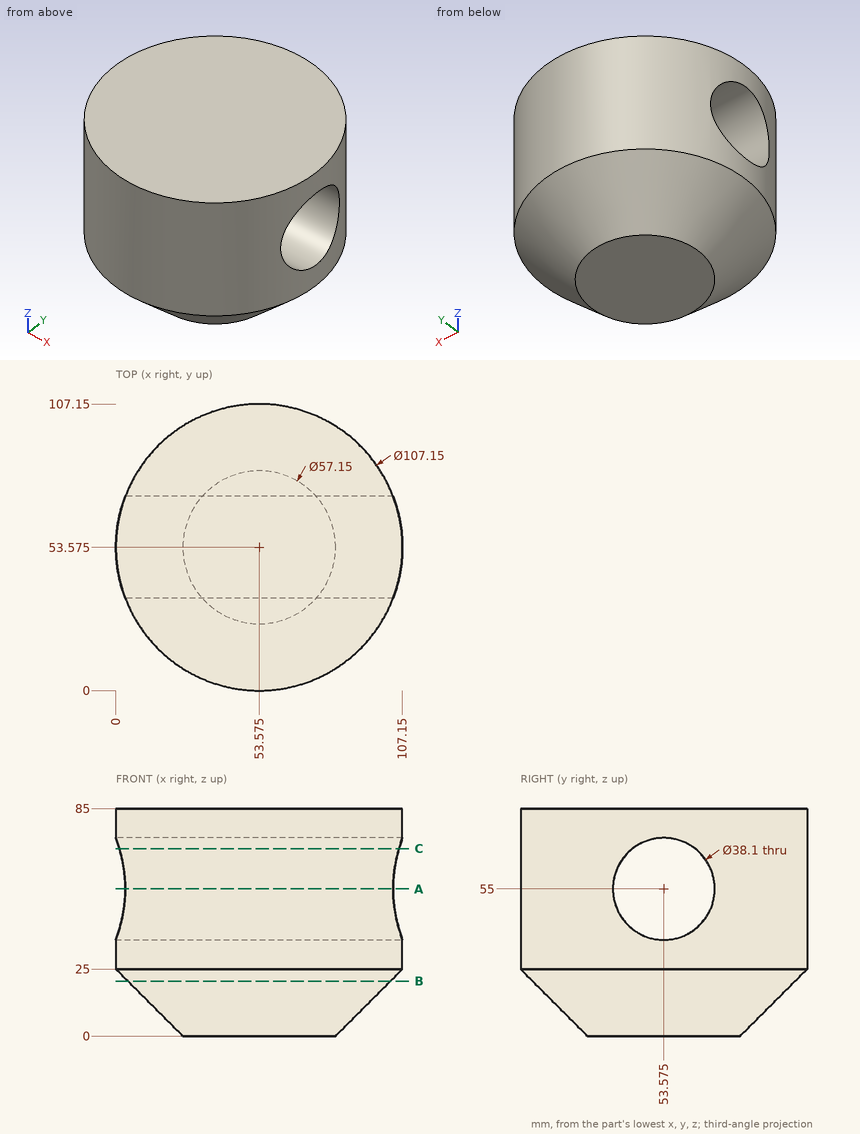
The figure shows three views and two pictorial views of one solid part (mm, origin at its lowest corner). Answer the questions. Coordinates: 2 decimals unless noted, no trailing zeros. Loops run counter-clockwise (first coordinate to the right, second up) from the corner with the lowest first, then second, coordinate; pieces in that order, holes last. Notation, with made-up numbers: M -12.75,20.25 L 18.25,20.25 A20 cw 18.25,44.25 Z; hole C 69,59 d11. An arc over 180 degrees is marked long. Use CSV: the item, a comma, the result in double quotes. Start each with the question number.
(1) Given pin 1 Ø2 at (x, z) = (95, 65.5) entering from +Y; pin 2 Ø1.5 at (y, z) = (37, 70) entering from -X; pin 3 Ø3 at (x, z) = (91, 16.5) entering from +Y; pin 4 Ø1 at (y, z) = (59, 38) entering from -X, each flat-ended and moving along its own axis, determine where each tip first touches the part or whether it passes through.
(2) Find section C-C, the plane z = 70. Give the vertices of the cut face in (x, y) (3 decimals), then the cut area to 3 significant figures.
(3) Find section B-B, the plane z = 20.5. Give the vertices of the cut face in (x, y) (3 decimals), then the cut area to 3 significant figures.
(4) Find section A-A, the plane z = 55. Give the vertices of the cut face in (x, y) (3 decimals), then the cut area to 3 significant figures.
(5) Consider line 1 (Y direction, x = 38, z = 55) (3 decimals); line 2 (Y direction, x = 101.5, z = 56); line 3 (Z direction, x = 12.5, y = 54). Determine where each line is inside the solid, lowest interval first.
Recorded:
1,pin 1,"stops at y = 88.73"
1,pin 2,"stops at x = 2.39"
1,pin 3,"stops at y = 81.99"
1,pin 4,"passes through"
2,outline,"M 1.303,41.832 A53.575 ccw 105.847,41.832 Z; M 1.303,65.318 L 105.847,65.318 A53.575 ccw Z"
2,area,"6,520 mm^2"
3,outline,"C 53.575,53.575 d98.15"
3,area,"7,570 mm^2"
4,outline,"M 3.501,34.525 A53.575 ccw 103.649,34.525 Z; M 3.501,72.625 L 103.649,72.625 A53.575 ccw Z"
4,area,"5,020 mm^2"
5,line 1,"y = 2.314 to 34.525, 72.625 to 104.836"
5,line 2,"y = 29.63 to 34.55, 72.6 to 77.52"
5,line 3,"z = 12.5 to 35.95, 74.05 to 85"
